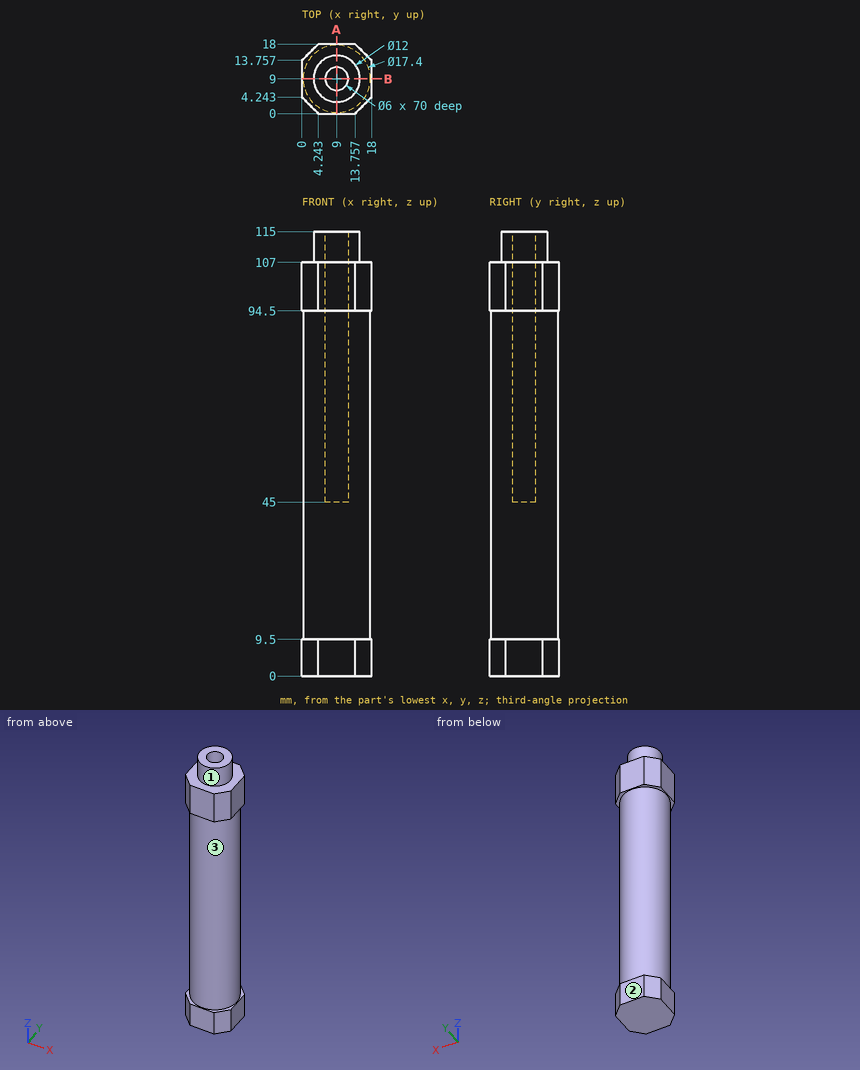
Answer from the drawing. Dimensions are ordinates in mm from the lowest x, y and z of the part. A direction names the side the tool comes from. Give positions to 0.01 mm unless a question says otherwise; leave off trailing zeros. Write each loop counter-clockwise with the first axis right and the second up, starting at its lowest first coordinate (ties: lowest second). Pieces come first, ordered by that corner, then holes. Notation, with made-up numbers: (-15, 25.5) - (30, 25.5) arc R17 cw to (30, 35.5) - close; hole circle Ø3 at (38.25, 30.25). An arc over 180 degrees is marked (long way). One line per item, written item: value. Start each with the question number.
1. Consider probe 1 along Y at (x, z) = (9, 73); probe 2 along Y at (x, z) = (9, 98); probe 3 along Z at (x, y) = (1.75, 14.5). Determine where each line is inside the solid, lowest interval first.
2. For the marked faces 1, 2 and 3, determine the directions among +Z, -Z, +X, -X, +Y, -Y from which every point of the face is accessible in a straight line to the end or side of a thin tool.
3. Find section A-A (x = 9). Write down the section's boundary in (y, z), then the cut area to 3 significant figures.
4. Given pin 1 (8 mm diameter, centred on y = 2.5, z = 46.5, fed in from -X); pin 2 (8 mm diameter, centred on y = 5, z = 70, fed in from +X); pin 3 (1 mm diameter, centred on x = 2.5, y = 10.5, fed in from +Z), each flat-ended and moving along its own axis, determine where each tip first touches the part or whether it passes through.
Geometry results:
1. probe 1: 0.3 to 6, 12 to 17.7
1. probe 2: 0 to 6, 12 to 18
1. probe 3: 0 to 9.5, 94.5 to 107
2. face 1: +Z
2. face 2: +Z, -Z, +X, -X, +Y
2. face 3: none
3. outline: (0, 0) - (18, 0) - (18, 9.5) - (17.7, 9.5) - (17.7, 94.5) - (18, 94.5) - (18, 107) - (15, 107) - (15, 115) - (12, 115) - (12, 45) - (6, 45) - (6, 115) - (3, 115) - (3, 107) - (0, 107) - (0, 94.5) - (0.3, 94.5) - (0.3, 9.5) - (0, 9.5) - close
3. area: 1,550 mm2
4. pin 1: x = 0.67
4. pin 2: x = 17.7
4. pin 3: z = 107
